For this review, take the finished solid that the model builds, in its own axes (mm). A direction names the side the tool comes from. Give positions to 0.01 mm unless a question says otherwise; leave off trailing zeros. Order: outer loops, then holes, each group sorted by start corner. A loop starts at its lowest first (then second) coordinate and runs counter-clockwise, first axis right, second up. Notation, with made-up numbers: (-6, 4.25) -> (31, 4.25) arc R21 cw to (31, 29.25) -> close; hole circle Ø7 at (10, -16.5). An arc over 180 degrees is marked (long way). Return JSON: item names as keys, results as strings. Group by question number.
1) Add section D-D (y = 54.5). Give the boundary of the cut face in (x, z), then the cut area to 3 significant figures.
2) Add section A-A (x = -30). Give the boundary of the cut face in (y, z), then the cut area to 3 significant figures.
3) Add section B-B (z = 2.3). Give the boundary of the cut face in (x, y), then the cut area to 3 significant figures.
4) The part is to be moulded in two halves that separate along X. For faces 3 (the face through (-11, 1, 3)), 4 (the face through (-47, 1, 1)), 5 (the face through (-42.474, 53.148, 1.986)), say which applies: released by +X, released by -X, zero draft, split by the parting line, or undercut.
5) For faces 1 (the face through (-9, 1, 1)), 2 (the face through (-1, -62.5, 1)), list the 3-axis set-ups (+Z, -Z, +X, -X, +Y, -Y) from which the entire face can be reached by the end or side of a thin tool; tool diameter is ignored.
6) Insertion check: P1, Ø4, axis at x = -17, y = 18, coming from the -Z side; P2, Ø3.5, axis at x = 41, y = 54.5, coming from the +Z side (1 decimal). Each pin has a flat end and moves straight along its axis. Give the tip position at first contact, or say it passes through.
7) Add section C-C (x = -41). Give the boundary of the cut face in (y, z).
8) To check wall thickness, follow line 1 along Y through (x, z) = (-41, 1.9); line 2 along X through (y, z) = (-45.5, 1.7); line 3 along X through (y, z) = (13, 1.1). State the ranges of each line that lie inside material, in increasing order.
Autodesk Inventor part; units mm, degrees
ref_plane "Piano di lavoro1" through (0, 0, 0) normal (0, 0, 1) x (1, 0, 0)
ref_plane "YZ Plane" through (0, 0, 0) normal (1, 0, 0) x (0, 1, 0)
ref_plane "XZ Plane" through (0, 0, 0) normal (0, 1, 0) x (-1, 0, 0)
ref_plane "Piano di lavoro1" through (0, 0, 0) normal (0, 0, 1) x (1, 0, 0)
sketch "Schizzo1" plane through (0, 0, 0) normal (0, 0, 1) x (1, 0, 0)
  line L0 (16, 20.5) -> (-6, 20.5)
  line L1 (16, -9.5) -> (16, 20.5)
  line L2 (-6, -9.5) -> (16, -9.5)
  line L3 (-6, 20.5) -> (-6, -9.5)
  line L4 (-21, 10.5) -> (-21, 28.5)
  line L5 (-21, 28.5) -> (-36, 28.5)
  line L6 (-36, 10.5) -> (-21, 10.5)
  line L7 (-36, 28.5) -> (-36, 10.5)
  circle A0 centre (-41, 54.5) radius 2
  circle A1 centre (41, 54.5) radius 2
  circle A2 centre (41, -45.5) radius 2
  circle A3 centre (-41, -45.5) radius 2
  line L8 (47, -62.5) -> (-47, -62.5)
  line L9 (47, 62.5) -> (47, -62.5)
  line L10 (-47, 62.5) -> (47, 62.5)
  line L11 (-47, -62.5) -> (-47, 62.5)
  point P0 (0, 0)
extrude "Estrusione1" add sketch "Schizzo1" along normal blind 2
sketch "Schizzo2" plane through (0, 0, 0) normal (0, 0, -1) x (-1, 0, 0)
  line L0 (-47, -62.5) -> (-47, 62.5)
  line L1 (47, -62.5) -> (-47, -62.5)
  line L2 (47, 62.5) -> (47, -62.5)
  line L3 (-47, 62.5) -> (47, 62.5)
  circle A0 centre (41, 54.5) radius 2
  circle A1 centre (-41, 54.5) radius 2
  circle A2 centre (-41, -45.5) radius 2
  circle A3 centre (41, -45.5) radius 2
  line L4 (6, -9.5) -> (6, 20.5)
  line L5 (-16, -9.5) -> (6, -9.5)
  line L6 (-16, 20.5) -> (-16, -9.5)
  line L7 (6, 20.5) -> (-16, 20.5)
  line L8 (36, 10.5) -> (36, 28.5)
  line L9 (21, 10.5) -> (36, 10.5)
  line L10 (21, 28.5) -> (21, 10.5)
  line L11 (36, 28.5) -> (21, 28.5)
  point P0 (0, 0)
sketch "Schizzo3" plane through (0, 0, 0) normal (0, 0, -1) x (-1, 0, 0)
  line L0 (45, 60.5) -> (-45, 60.5)
  line L1 (-45, 60.5) -> (-45, -60.5)
  line L2 (45, -60.5) -> (45, 60.5)
  line L3 (-45, -60.5) -> (45, -60.5)
  point P0 (0, 0)
extrude "Estrusione2" cut sketch "Schizzo3" against normal blind 1
sketch "Schizzo4" plane through (-47, -62.5, 0) normal (0, -1, 0) x (1, 0, 0)
  line L0 (0, 0) -> (94, 0)
  line L1 (94, 0) -> (94, 2)
  line L2 (0, 2) -> (94, 2)
  line L3 (0, 0) -> (0, 2)
  line L4 (0, 0) -> (94, 0)
  line L5 (94, 0) -> (94, 2)
  line L6 (0, 2) -> (94, 2)
  line L7 (0, 0) -> (0, 2)
  point P0 (47, 0)
sketch "Schizzo5" plane through (0, 0, 2) normal (0, 0, 1) x (1, 0, 0)
  line L0 (47, -62.5) -> (47, 62.5)
  line L1 (47, 62.5) -> (-47, 62.5)
  line L2 (-47, 62.5) -> (-47, -62.5)
  line L3 (-47, -62.5) -> (47, -62.5)
  circle A0 centre (-41, 54.5) radius 2
  circle A1 centre (41, 54.5) radius 2
  circle A2 centre (41, -45.5) radius 2
  circle A3 centre (-41, -45.5) radius 2
  line L4 (-6, -9.5) -> (-6, 20.5)
  line L5 (-6, 20.5) -> (16, 20.5)
  line L6 (16, 20.5) -> (16, -9.5)
  line L7 (16, -9.5) -> (-6, -9.5)
  line L8 (-36, 10.5) -> (-36, 28.5)
  line L9 (-36, 28.5) -> (-21, 28.5)
  line L10 (-21, 28.5) -> (-21, 10.5)
  line L11 (-21, 10.5) -> (-36, 10.5)
  point P0 (0, 0)
extrude "Estrusione3" add sketch "Schizzo5" along normal blind 1
properties part number "_Stampa 3D"
Evaluation:
{
 "1": {"outline": "(-47, 0) -> (-45, 0) -> (-45, 1) -> (-43, 1) -> (-43, 3) -> (-47, 3) -> close; (-39, 1) -> (39, 1) -> (39, 3) -> (-39, 3) -> close; (43, 1) -> (45, 1) -> (45, 0) -> (47, 0) -> (47, 3) -> (43, 3) -> close", "area": "176 mm^2"},
 "2": {"outline": "(-62.5, 0) -> (-60.5, 0) -> (-60.5, 1) -> (10.5, 1) -> (10.5, 3) -> (-62.5, 3) -> close; (28.5, 1) -> (60.5, 1) -> (60.5, 0) -> (62.5, 0) -> (62.5, 3) -> (28.5, 3) -> close", "area": "218 mm^2"},
 "3": {"outline": "(-47, -62.5) -> (47, -62.5) -> (47, 62.5) -> (-47, 62.5) -> close; hole circle Ø4 at (-41, -45.5); hole circle Ø4 at (-41, 54.5); hole (-36, 10.5) -> (-21, 10.5) -> (-21, 28.5) -> (-36, 28.5) -> close; hole (-6, -9.5) -> (16, -9.5) -> (16, 20.5) -> (-6, 20.5) -> close; hole circle Ø4 at (41, -45.5); hole circle Ø4 at (41, 54.5)", "area": "10,800 mm^2"},
 "4": {"face 3": "zero draft", "face 4": "released by -X", "face 5": "undercut"},
 "5": {"face 1": "-Z", "face 2": "+Z, -Z, +X, -X, -Y"},
 "6": {"P1": "z = 1", "P2": "through"},
 "7": {"outline": "(-62.5, 0) -> (-60.5, 0) -> (-60.5, 1) -> (-47.5, 1) -> (-47.5, 3) -> (-62.5, 3) -> close; (-43.5, 1) -> (52.5, 1) -> (52.5, 3) -> (-43.5, 3) -> close; (56.5, 1) -> (60.5, 1) -> (60.5, 0) -> (62.5, 0) -> (62.5, 3) -> (56.5, 3) -> close"},
 "8": {"line 1": "-62.5 to -47.5, -43.5 to 52.5, 56.5 to 62.5", "line 2": "-47 to -43, -39 to 39, 43 to 47", "line 3": "-47 to -36, -21 to -6, 16 to 47"}
}
